Can you work these out from the model? Positions are in its coordinate system, mm. A direction names the side the tool comes from. Coordinates: 2 decimals unless noted, no trailing zeros. Write each loop counter-clockwise with the first axis right and the second up, starting at its lowest first coordinate (ties: lowest second). Pieces come first, ordered by that corner, then holes. Notation, with made-up numbers: M 33.5,69.5 L 67.5,69.5 A19 ccw 67.5,103.5 Z; hole C -4.5,22 d2. An arc over 180 degrees is marked long. Use one line per item in the form item = value. Start each with the question number.
```python
from build123d import *

# Parameters (mm, degrees)
REVOLUTION004_FACE6_R = 23.05
PAD006_DEPTH          = 10
PAD007_DEPTH          = 2
PAD008_DEPTH          = 2


with BuildPart() as part:
    # Sketch016 → Revolution003 (revolve)
    with BuildSketch(Plane.YZ):
        Polygon((19.625, -22.587589), (19.625, 0), (16.75, 0), (16.75, -24.1609), (17.75, -24.1609), align=None)
    revolve(axis=Axis((0, 0, 0), (0, 0, 1)))

    # Export → Loft section 0
    with BuildSketch(Plane.XY):
        with BuildLine():
            ThreePointArc((7.510162, 18.131136), (0, 19.625), (-7.510162, 18.131136))
            ThreePointArc((-7.510162, 18.131136), (-13.876971, 13.876971), (-18.131136, 7.510162))
            ThreePointArc((-18.131136, 7.510162), (-19.625, 0), (-18.131136, -7.510162))
            ThreePointArc((-18.131136, -7.510162), (-13.876971, -13.876971), (-7.510162, -18.131136))
            ThreePointArc((-7.510162, -18.131136), (0, -19.625), (7.510162, -18.131136))
            ThreePointArc((7.510162, -18.131136), (13.876971, -13.876971), (18.131136, -7.510162))
            ThreePointArc((18.131136, -7.510162), (19.625, 0), (18.131136, 7.510162))
            ThreePointArc((18.131136, 7.510162), (13.876971, 13.876971), (7.510162, 18.131136))
        make_face()
    # Export002 → Loft section 1
    with BuildSketch(Plane.XY.offset(50)):
        with BuildLine():
            Line((-50, 40), (-50, -40))
            ThreePointArc((-50, -40), (-47.071068, -47.071068), (-40, -50))
            Line((-40, -50), (40, -50))
            ThreePointArc((40, -50), (47.071068, -47.071068), (50, -40))
            Line((50, -40), (50, 40))
            ThreePointArc((50, 40), (47.071068, 47.071068), (40, 50))
            Line((40, 50), (-40, 50))
            ThreePointArc((-40, 50), (-47.071068, 47.071068), (-50, 40))
        make_face()
    loft()

    # Sketch020 → Revolution004 (revolve)
    with BuildSketch(Plane.YZ):
        Polygon((23.05, 0), (16.75, 0), (16.75, -5), (19.625, -5), (23.05, -5), align=None)
    revolve(axis=Axis((0, 0, 0), (0, 0, 1)))

    # Revolution004 Face6 → Pad006 (new)
    with BuildSketch(Plane(origin=(0, 0, 0), x_dir=(0, 1, 0), z_dir=(0, 0, 1))):
        Circle(REVOLUTION004_FACE6_R)
        with BuildLine():
            ThreePointArc((19.625, 0), (19.247911, -3.828648), (18.131136, -7.510162))
            ThreePointArc((18.131136, -7.510162), (13.876971, -13.876971), (7.510162, -18.131136))
            ThreePointArc((7.510162, -18.131136), (0, -19.625), (-7.510162, -18.131136))
            ThreePointArc((-7.510162, -18.131136), (-13.876971, -13.876971), (-18.131136, -7.510162))
            ThreePointArc((-18.131136, -7.510162), (-19.625, 0), (-18.131136, 7.510162))
            ThreePointArc((-18.131136, 7.510162), (-13.876971, 13.876971), (-7.510162, 18.131136))
            ThreePointArc((-7.510162, 18.131136), (0, 19.625), (7.510162, 18.131136))
            ThreePointArc((7.510162, 18.131136), (13.876971, 13.876971), (18.131136, 7.510162))
            ThreePointArc((18.131136, 7.510162), (19.247911, 3.828648), (19.625, 0))
        make_face(mode=Mode.SUBTRACT)
    extrude(amount=PAD006_DEPTH)

    # Export003 → Loft001 section 0
    with BuildSketch(Plane.XY):
        with BuildLine():
            ThreePointArc((6.409947, 15.474982), (0, 16.75), (-6.409947, 15.474982))
            ThreePointArc((-6.409947, 15.474982), (-11.844039, 11.844039), (-15.474982, 6.409947))
            ThreePointArc((-15.474982, 6.409947), (-16.75, 0), (-15.474982, -6.409947))
            ThreePointArc((-15.474982, -6.409947), (-11.844039, -11.844039), (-6.409947, -15.474982))
            ThreePointArc((-6.409947, -15.474982), (0, -16.75), (6.409947, -15.474982))
            ThreePointArc((6.409947, -15.474982), (11.844039, -11.844039), (15.474982, -6.409947))
            ThreePointArc((15.474982, -6.409947), (16.75, 0), (15.474982, 6.409947))
            ThreePointArc((15.474982, 6.409947), (11.844039, 11.844039), (6.409947, 15.474982))
        make_face()
    # Export004 → Loft001 section 1
    with BuildSketch(Plane.XY.offset(50)):
        with BuildLine():
            Line((-47, 40), (-47, -40))
            ThreePointArc((-47, -40), (-44.949747, -44.949747), (-40, -47))
            Line((-40, -47), (40, -47))
            ThreePointArc((40, -47), (44.949747, -44.949747), (47, -40))
            Line((47, -40), (47, 40))
            ThreePointArc((47, 40), (44.949747, 44.949747), (40, 47))
            Line((40, 47), (-40, 47))
            ThreePointArc((-40, 47), (-44.949747, 44.949747), (-47, 40))
        make_face()
    loft(mode=Mode.SUBTRACT)

    # Loft001 Face13 → Pad007 (add)
    with BuildSketch(Plane(origin=(0, 0, 50), x_dir=(0, 1, 0), z_dir=(0, 0, 1))):
        with BuildLine():
            Line((40, 50), (-40, 50))
            ThreePointArc((-40, 50), (-47.071068, 47.071068), (-50, 40))
            Line((-50, 40), (-50, -40))
            ThreePointArc((-50, -40), (-47.071068, -47.071068), (-40, -50))
            Line((-40, -50), (40, -50))
            ThreePointArc((40, -50), (47.071068, -47.071068), (50, -40))
            Line((50, -40), (50, 40))
            ThreePointArc((50, 40), (47.071068, 47.071068), (40, 50))
        make_face()
        with BuildLine():
            Line((47, 40), (47, -40))
            ThreePointArc((47, -40), (44.949747, -44.949747), (40, -47))
            Line((40, -47), (-40, -47))
            ThreePointArc((-40, -47), (-44.949747, -44.949747), (-47, -40))
            Line((-47, -40), (-47, 40))
            ThreePointArc((-47, 40), (-44.949747, 44.949747), (-40, 47))
            Line((-40, 47), (40, 47))
            ThreePointArc((40, 47), (44.949747, 44.949747), (47, 40))
        make_face(mode=Mode.SUBTRACT)
    extrude(amount=PAD007_DEPTH)

    # Sketch019 (on Sketch) → Pad008 (join)
    with BuildSketch(Plane.XY.offset(50)):
        with BuildLine():
            ThreePointArc((50, 55), (47.071068, 62.071068), (40, 65))
            Line((40, 65), (-55, 65))
            ThreePointArc((-55, 65), (-62.071068, 62.071068), (-65, 55))
            Line((-65, 55), (-65, -40))
            ThreePointArc((-65, -40), (-62.071068, -47.071068), (-55, -50))
            Line((-55, -50), (-40, -50))
            Line((-40, -50), (-40, -47))
            ThreePointArc((-40, -47), (-44.949747, -44.949747), (-47, -40))
            Line((-47, -40), (-47, 40))
            ThreePointArc((-47, 40), (-44.949747, 44.949747), (-40, 47))
            Line((-40, 47), (40, 47))
            ThreePointArc((40, 47), (44.949747, 44.949747), (47, 40))
            Line((47, 40), (50, 40))
            Line((50, 40), (50, 55))
        make_face()
    extrude(amount=PAD008_DEPTH)


solid = part.part
```
1) Suppose I cut it at A-A on z = -6.5. Please give me the cut outline in (x, y) (3 decimals), and give its area (3 significant figures).
2) Which directions (+Z, -Z, +X, -X, +Y, -Y) give clear straight access to the entire face, cutting with the end or side of a thin tool? Please do faces 1 (the face through (-45, 44.9, 51)), 2 (the face through (-11, -13, -24.161)), 3 (the face through (-10.4, -17, -5)).
3) If we mould it in two halves opening along Y, with no side actions, what happens to faces 4 (the face through (16.35, -3.63, -12.25)), 5 (the face through (47.15, 61.99, 50.99)), 6 (the face through (17.442, -3.873, -24.062)), 7 (the face through (-50.4, 24.8, 50))? For each: +Y half, -Y half, draft (parallel to the pull), parting line (faces both ways), or undercut.
4) Will these pins go through, and if not, where does the flat tip stop? pin 1 Ø8 at (x, y) = (37.5, -33.5) entering from +Z; pin 2 Ø3 at (y, z) = (-23.5, 28.5) entering from +X; pin 3 Ø4 at (x, z) = (-2, 11.5) entering from -Y; pin 4 Ø14 at (x, y) = (9.5, 9) entering from -Z.
5) Please list where these lines run through material, in increasing order: line 1 (Y direction, x = 0, z = -7) (3 decimals); line 2 (Z direction, x = -57.5, y = 42).
6) Suppose I cut it at B-B on y = 58.5. Please give me the cut outline in (x, z), and give its area (3 significant figures).
Computed values:
q1.outline = C 0,0 d39.25; hole C 0,0 d33.5
q1.area = 329 mm²
q2.face_1 = +Z
q2.face_2 = -Z, +X, -X, +Y, -Y
q2.face_3 = -Z
q3.face_4 = undercut
q3.face_5 = +Y half
q3.face_6 = parting line
q3.face_7 = draft
q4.pin_1 = 41.26
q4.pin_2 = 37.4
q4.pin_3 = -27.81
q4.pin_4 = -24.16
q5.line_1 = -19.625 to -16.75, 16.75 to 19.625
q5.line_2 = 50 to 52
q6.outline = M -64.37,50 L 49.37,50 L 49.37,52 L -64.37,52 Z
q6.area = 227 mm²
